Can you work these out from the model? Positions are in its coordinate system, mm. A direction names the side the tool comes from. Give positions to 0.01 mm unless a question says otherwise; leave off trailing zeros. Order: outer loops, then holes, each group sorted by start corner. A loop starts at its lowest first (then second) coordinate and runs counter-clockwise, first axis right, second up. Notation, with made-up numbers: M 69.25,32.5 L 97.25,32.5 A15 cw 97.25,38.5 Z; hole C 41,24.5 d2. An arc over 180 degrees is marked long. One line per question, with ' | ' between items. Start each with the question number.
1) Please list where these lines run through material, in increasing order: line 1 along X through (y, z) = (22.7, 6); line 2 along Y through (x, z) = (26.5, 30); line 3 along X through (y, z) = (13.5, 32). Write a range as [from, to].
2) If we section it at D-D, the plane z = 6: Please give me the cut outline in (x, y), plus the area to 3 significant figures.
3) For faces 4 (the flat face through (44, 12, 30.35)), 5 (the flat face through (20, 22.3, 20)), 6 (the cylindrical face through (42.465, 6.996, 35.597)), 7 (the flat face through (47.4, 20, 36)), which set-ups out of +Z, -Z, +X, -X, +Y, -Y let a thin tool reach every point of the face, with its end or its side?
4) If we section it at B-B, the plane z = 13: Please give me the cut outline in (x, y), plus the area to 3 significant figures.
5) If we section it at C-C, the plane x = 49.1: Please give me the cut outline in (y, z).
6) I'm going to push flat-ended pins straight in: pin 1 Ø1.9 at (x, z) = (49.1, 28) entering from -Y; pin 2 Ø1.2 at (y, z) = (4.5, 33) entering from -X; pin 3 Ø2 at (x, y) = (-3.5, 8.5) entering from -Z; pin 4 Ø1.5 at (x, y) = (37, 6) entering from -Z. Where does each tip first touch, or does it pass through?
7) Thinking about a two-plate mould opening in Z: for faces 1 (the flat face through (20, 2, 20)), 2 (the flat face through (20, 1, 0)), 3 (the cylindrical face through (50.45, 1.01, 6.86)), which applies, +Z half, -Z half, draft (parallel to the pull), parting line (faces both ways), or undercut?
8) If we section it at A-A, the plane y = 12.15: Please give me the cut outline in (x, z), plus the area to 3 significant figures.
```python
from build123d import *

# Parameters (mm, degrees)
SKETCH1_W             = 40.2
SKETCH1_H             = 2
BOSS_EXTRUDE1_DEPTH   = 40.7
BOSS_EXTRUDE1_2_DEPTH = 40.7
BOSS_EXTRUDE3_START   = 40.7
SKETCH1_3_R           = 6.6
BOSS_EXTRUDE3_DEPTH   = 1
BOSS_EXTRUDE2_START   = -1
BOSS_EXTRUDE2_DEPTH   = 10.35
SKETCH4_R             = 1.6
BOSS_EXTRUDE4_DEPTH   = 2
BOSS_EXTRUDE5_START   = -22.3
SKETCH4_3_W           = 70
SKETCH4_3_H           = 40.7
SKETCH4_3_R           = 1.6
BOSS_EXTRUDE5_DEPTH   = 2


with BuildPart() as part:
    # Sketch1 → Boss-Extrude1 (new body)
    with BuildSketch(Plane.XY):
        with Locations((20.1, 23.3)):
            Rectangle(SKETCH1_W, SKETCH1_H)
    extrude(amount=BOSS_EXTRUDE1_DEPTH)



with BuildPart() as body_2:
    # Sketch1 → Boss-Extrude1 2 (new body)
    with BuildSketch(Plane.XY):
        Polygon((0, 2), (0, 0), (40.2, 0), (40.2, 2), (40.1, 2), (0.1, 2), align=None)
    extrude(amount=BOSS_EXTRUDE1_2_DEPTH)


with BuildPart() as part_1:
    add(part.part)

    add(body_2.part)  # Boss-Extrude3 merges body 2
    # Sketch1<3> → Boss-Extrude3 (add)
    with BuildSketch(Plane.XY.offset(BOSS_EXTRUDE3_START)):
        Polygon((0, 22.3), (0, 2), (0.1, 2), (40.1, 2), (40.2, 2), (40.2, 22.3), align=None)
        with Locations((9.7, 12.15)):
            Circle(SKETCH1_3_R, mode=Mode.SUBTRACT)
    extrude(amount=-BOSS_EXTRUDE3_DEPTH)

    # Sketch3 → Boss-Extrude2 (add)
    with BuildSketch(Plane(origin=(0, -15.7, 39.7), x_dir=(1, 0, 0), z_dir=(0, 0, -1)).offset(BOSS_EXTRUDE2_START)):
        with BuildLine():
            ThreePointArc((-6.315, -21.675), (-2.26366714, -22.775), (-6.315, -23.875))
            Line((-6.315, -23.875), (-7.2, -23.875))
            Line((-7.2, -23.875), (-7.2, -31.825))
            Line((-7.2, -31.825), (-6.315, -31.825))
            ThreePointArc((-6.315, -31.825), (-2.26366714, -32.925), (-6.315, -34.025))
            Line((-6.315, -34.025), (-7.2, -34.025))
            Line((-7.2, -34.025), (-7.2, -40))
            Line((-7.2, -40), (0, -40))
            Line((0, -40), (0, -15.7))
            Line((0, -15.7), (-7.2, -15.7))
            Line((-7.2, -15.7), (-7.2, -21.675))
            Line((-7.2, -21.675), (-6.315, -21.675))
        make_face()
    boss_extrude2 = extrude(amount=BOSS_EXTRUDE2_DEPTH)

    # Mirror1: Boss-Extrude2 across plane
    add(boss_extrude2.mirror(Plane(origin=(20.1, 0, 0), x_dir=(0, 0, 1), z_dir=(1, 0, 0))))

    # Sketch4 → Boss-Extrude4 (add)
    # profile 1 of 2: a face of its own
    with BuildSketch(Plane(origin=(0, 24.3, 0), x_dir=(1, 0, 0), z_dir=(0, 1, 0))):
        Polygon((0, 0), (-14.9, 0), (-14.9, -40.7), (-7.2, -40.7), (-7.2, -30.35), (0, -30.35), align=None)
        with Locations(Location((-8.9, -28, 0), (0, 0, 270))):
            Circle(SKETCH4_R, mode=Mode.SUBTRACT)
        with Locations(Location((-8.9, -6, 0), (0, 0, 270))):
            Circle(SKETCH4_R, mode=Mode.SUBTRACT)
    # profile 2 of 2: a face of its own
    with BuildSketch(Plane(origin=(0, 24.3, 0), x_dir=(1, 0, 0), z_dir=(0, 1, 0))):
        Polygon((55.1, 0), (40.2, 0), (40.2, -30.35), (47.4, -30.35), (47.4, -40.7), (55.1, -40.7), align=None)
        with Locations(Location((49.1, -28, 0), (0, 0, 270))):
            Circle(SKETCH4_R, mode=Mode.SUBTRACT)
        with Locations(Location((49.1, -6, 0), (0, 0, 270))):
            Circle(SKETCH4_R, mode=Mode.SUBTRACT)
    extrude(amount=-BOSS_EXTRUDE4_DEPTH)

    # Sketch4<3> → Boss-Extrude5 (add)
    with BuildSketch(Plane(origin=(0, 24.3, 0), x_dir=(1, 0, 0), z_dir=(0, 1, 0)).offset(BOSS_EXTRUDE5_START)):
        with Locations((20.1, -20.35)):
            Rectangle(SKETCH4_3_W, SKETCH4_3_H)
        with Locations(Location((-8.9, -6, 0), (0, 0, 270))):
            Circle(SKETCH4_3_R, mode=Mode.SUBTRACT)
        with Locations(Location((49.1, -6, 0), (0, 0, 270))):
            Circle(SKETCH4_3_R, mode=Mode.SUBTRACT)
        with Locations(Location((49.1, -28, 0), (0, 0, 270))):
            Circle(SKETCH4_3_R, mode=Mode.SUBTRACT)
        with Locations(Location((-8.9, -28, 0), (0, 0, 270))):
            Circle(SKETCH4_3_R, mode=Mode.SUBTRACT)
    extrude(amount=-BOSS_EXTRUDE5_DEPTH)


solid = part_1.part
```
Results found:
1) line 1: x = [-14.9, -10.5], [-7.3, 47.5], [50.7, 55.1] | line 2: y = [0, 2], [22.3, 24.3] | line 3: x = [-7.2, 0], [40.2, 47.4]
2) outline: M -14.9,0 L -10.5,0 L -10.5,2 L -14.9,2 Z; M -14.9,22.3 L -10.5,22.3 L -10.5,24.3 L -14.9,24.3 Z; M -7.3,0 L 47.5,0 L 47.5,2 L -7.3,2 Z; M -7.3,22.3 L 47.5,22.3 L 47.5,24.3 L -7.3,24.3 Z; M 50.7,0 L 55.1,0 L 55.1,2 L 50.7,2 Z; M 50.7,22.3 L 55.1,22.3 L 55.1,24.3 L 50.7,24.3 Z | area: 254 mm²
3) face 4: -Z, +X, -X | face 5: -Z | face 6: +Z, -Z | face 7: +Z, -Z, +X
4) outline: M -14.9,0 L 55.1,0 L 55.1,2 L -14.9,2 Z; M -14.9,22.3 L 55.1,22.3 L 55.1,24.3 L -14.9,24.3 Z | area: 280 mm²
5) outline: M 0,0 L 2,0 L 2,4.4 L 0,4.4 Z; M 0,7.6 L 2,7.6 L 2,26.4 L 0,26.4 Z; M 0,29.6 L 2,29.6 L 2,40.7 L 0,40.7 Z; M 22.3,0 L 24.3,0 L 24.3,4.4 L 22.3,4.4 Z; M 22.3,7.6 L 24.3,7.6 L 24.3,26.4 L 22.3,26.4 Z; M 22.3,29.6 L 24.3,29.6 L 24.3,40.7 L 22.3,40.7 Z
6) pin 1: passes through | pin 2: stops at x = -7.2 | pin 3: stops at z = 30.35 | pin 4: stops at z = 39.7
7) face 1: draft | face 2: -Z half | face 3: undercut
8) outline: M -7.2,30.35 L 0,30.35 L 0,39.7 L 3.1,39.7 L 3.1,40.7 L -7.2,40.7 Z; M 16.3,39.7 L 40.2,39.7 L 40.2,30.35 L 47.4,30.35 L 47.4,40.7 L 16.3,40.7 Z | area: 176 mm²
